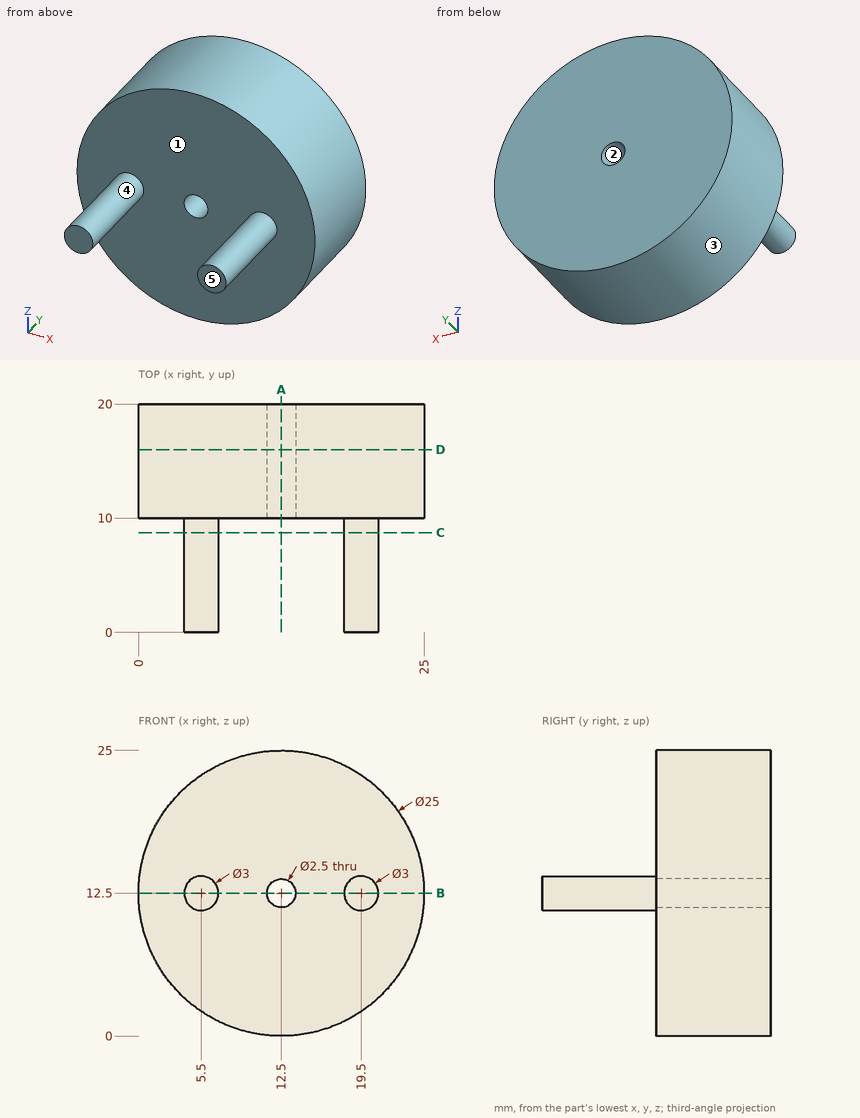
Job drawing, mm, ordinate dimensions from the low corner. One solid piece. A direction names the side the tool comes from. Round coordinates to 2 decimals unless told otherwise and drop trailing zeros. Write each loop counter-clockwise with the first axis right and the second up, starting at its lowest first coordinate (ties: lowest second). Pieces come first, ordered by that corner, then holes.
1) Band-saw the part on D-D, the plane y = 16. List the corners of the cut face in (x, z), and give its area (3 significant figures).
2) Band-saw the part on A-A, the plane x = 12.5. List the corners of the cut face in (y, z).
3) Band-saw the part on C-C, the plane y = 8.75. List the corners of the cut face in (x, z), and give its area (3 significant figures).
4) Band-saw the part on B-B, the plane z = 12.5. List the corners of the cut face in (x, y), and give its area (3 significant figures).
5) Pin check, flat tips, straight feed: pin 1 (8 mm diameter, centred on y = 13, z = 3, fed in from -X) (3 decimals); pin 2 (1.5 mm diameter, centred on x = 7, z = 9.5, fed in from -Y); pin 3 (12 mm diameter, centred on x = 12.5, y = 2, fed in from -Z). Stop position of each tip, or through.
6) Drill centre lines: probe 1 along Z at (x, y) = (12.5, 15.75); probe 2 along Y at (x, z) = (20, 18.75); probe 3 along X at (y, z) = (12.75, 5.5). Where is each one in solid material? Low to high.
7) 3-axis set-ups, long thin cutter, end or side, ignore diameter. For the marked faces 4 and 5: which of +Z, -Z, +X, -X, +Y, -Y reach the whole face in a straight line?
8) Mould opens along Z. For the marked faces 1, 2 and 3 say: +Z half, -Z half, draft (parallel to the pull), parting line (faces both ways), or undercut.
Ans:
1. outline: circle Ø25 at (12.5, 12.5); hole circle Ø2.5 at (12.5, 12.5)
1. area: 486 mm2
2. outline: (10, 0) - (20, 0) - (20, 11.25) - (10, 11.25) - close; (10, 13.75) - (20, 13.75) - (20, 25) - (10, 25) - close
3. outline: circle Ø3 at (5.5, 12.5); circle Ø3 at (19.5, 12.5)
3. area: 14.1 mm2
4. outline: (0, 10) - (4, 10) - (4, 0) - (7, 0) - (7, 10) - (11.25, 10) - (11.25, 20) - (0, 20) - close; (13.75, 10) - (18, 10) - (18, 0) - (21, 0) - (21, 10) - (25, 10) - (25, 20) - (13.75, 20) - close
4. area: 285 mm2
5. pin 1: stops at x = 1.275
5. pin 2: stops at y = 10
5. pin 3: stops at z = 11.38
6. probe 1: z = 0 to 11.25, 13.75 to 25
6. probe 2: y = 10 to 20
6. probe 3: x = 2.14 to 22.86
7. face 4: -Y
7. face 5: +Z, -Z, +X, -X, -Y
8. face 1: draft
8. face 2: undercut
8. face 3: parting line
